Here's the drawing with two shaded views (mm, measured from the low corner). I have some questions. A direction names the side the tool comes from. Give positions to 0.01 mm unless a question says otherwise; leave off trailing zeros. Write each loop counter-clockwise with the first axis right and the second up, starting at its lowest first coordinate (ties: lowest second). Pieces come first, ordered by that corner, then holes. Notation, with made-up numbers: (42.5, 7) - (89.5, 7) arc R21 ccw to (89.5, 45) - close; hole circle Ø2 at (-3.75, 16.5). An arc over 180 degrees is marked (long way). Write item = value, one per line.
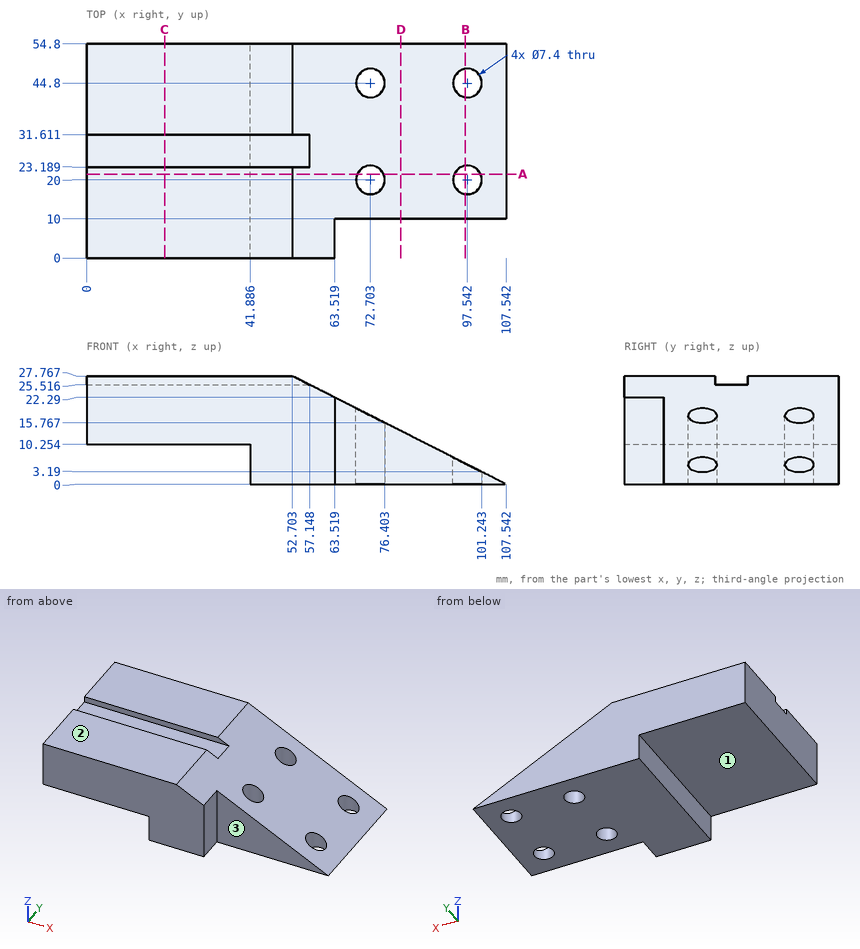
1. If we section it at C-C, the plane x = 20: Please give me the cut outline in (y, z) (1 decimal).
Filled sheet:
outline = (0, 10.3) - (54.8, 10.3) - (54.8, 27.8) - (31.6, 27.8) - (31.6, 25.5) - (23.2, 25.5) - (23.2, 27.8) - (0, 27.8) - close
2. If we section it at A-A, the plane y = 21.5: Count the separate pieces of the cut face and the enclosed holes in it, and give its area (3 significant figures).
Filled sheet:
separate_pieces = 3
enclosed_holes = 0
area = 1,640 mm2
3. I need wall thicknesses on line 1 (X direction, y = 20, z = 3.25) (1 decimal); line 2 (Y direction, x = 88, z = 4.75); line 3 (X direction, y = 44.8, z = 2.25) (1 decimal). Which ranges of each line are inside material? Lowest first, please.
Filled sheet:
line_1 = 41.9 to 69, 76.4 to 93.8
line_2 = 10 to 54.8
line_3 = 41.9 to 69, 76.4 to 93.8, 101.2 to 103.1
4. If we section it at D-D, the plane x = 80.5: Please give me the cut outline in (y, z).
Filled sheet:
outline = (10, 0) - (54.8, 0) - (54.8, 13.69) - (10, 13.69) - close
5. Which directions (+Z, -Z, +X, -X, +Y, -Y) give clear straight access to the entire face, cutting with the end or side of a thin tool? Please do the marked faces 1, 2 and 3.
Filled sheet:
face_1 = -Z, -X, +Y, -Y
face_2 = +Z, +X, -X, +Y, -Y
face_3 = +Z, -Z, +X, -Y
6. For pin 1 (5 mm diameter, centred on y = 5.5, z = 12.5, fed in from +X); pin 2 (8.5 mm diameter, centred on x = 97.54, y = 44.8, fed in from -Z); pin 3 (5 mm diameter, centred on x = 91, z = 6.5, fed in from -Y); pin 4 (2.5 mm diameter, centred on x = 16.5, y = 29.5, fed in from +Z), each with a flat end and sliding along its axis, tell me the tip position at first contact or that it passes through.
Filled sheet:
pin_1 = 63.52
pin_2 = 0
pin_3 = 10
pin_4 = 25.52
7. If we section it at B-B, the plane x = 97: Please give me the cut outline in (y, z), and give its area (3 significant figures).
Filled sheet:
outline = (10, 0) - (16.34, 0) - (16.34, 5.34) - (10, 5.34) - close; (23.66, 0) - (41.14, 0) - (41.14, 5.34) - (23.66, 5.34) - close; (48.46, 0) - (54.8, 0) - (54.8, 5.34) - (48.46, 5.34) - close
area = 161 mm2
